For this review, take the finished solid that the model builds, in its own axes (mm). Give positions to 0.01 mm unless a question says otherwise; leave off trailing zeros. Write each loop counter-clockwise with the first axis right and the second up, starting at its lowest first coordinate (ties: lowest second). Pieces come first, ordered by that corner, then holes. Notation, with made-up numbers: (-31, -25.75) -> (27, -25.75) arc R29 cw to (27, -2.75) -> close; hole circle Ø3 at (60.5, 7). An arc over 180 degrees is marked (long way). Write item = value, one per line.
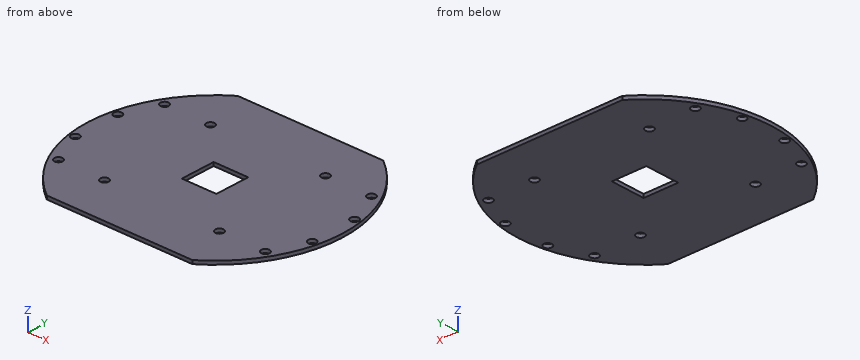
```python
from build123d import *

# Parameters (mm, degrees)
F1_DEPTH = 3
F3_D     = 7
F5_D     = 7
F6_W     = 30
F6_H     = 30
F7_DEPTH = 3.001


# Not quite as in the source:
# - a feature names something its author has since deleted; it is built from what else it names


with BuildPart() as f1:
    # F0 (on Top) → F1 (new body)
    with BuildSketch(Plane.XY):
        with BuildLine():
            Line((63.2455532034, 90), (-63.2455532034, 90))
            ThreePointArc((-63.2455532034, 90), (-110, 0), (-63.2455532034, -90))
            Line((-63.2455532034, -90), (63.2455532034, -90))
            ThreePointArc((63.2455532034, -90), (110, 0), (63.2455532034, 90))
        make_face()
    extrude(amount=F1_DEPTH)

    # F3 (through all)
    with Locations(Plane.XY.offset(3)):
        with Locations((-103, 20), (-103, -20), (-90, 50), (-90, -50), (90, -50), (90, 50), (103, 20), (103, -20)):
            Hole(F3_D / 2)

    # F5 (through all)
    with Locations(Plane.XY.offset(3)):
        with Locations((-50, 50), (50, 50), (50, -50), (-50, -50)):
            Hole(F5_D / 2)

    # F6 (on face) → F7 (cut, through all)
    with BuildSketch(Plane.XY.offset(3)):
        Rectangle(F6_W, F6_H)
    extrude(amount=-F7_DEPTH, mode=Mode.SUBTRACT)


solid = f1.part
```
(1) Take a section at B-B (x = 3.5). Write out the cut boundary in (y, z), plus the area to 3 significant figures.
Answers below:
outline = (-90, 0) -> (-15, 0) -> (-15, 3) -> (-90, 3) -> close; (15, 0) -> (90, 0) -> (90, 3) -> (15, 3) -> close
area = 450 mm^2
(2) Take a section at C-C (z = 0.85). Count the separate pieces of the cut face and the enclosed holes in it, plus the area to 3 significant figures.
Answers below:
separate_pieces = 1
enclosed_holes = 13
area = 33,200 mm^2
(3) Take a section at A-A (x = 90). Write out the cut boundary in (y, z), plus the area to 3 significant figures.
Answers below:
outline = (-63.25, 0) -> (-53.5, 0) -> (-53.5, 3) -> (-63.25, 3) -> close; (-46.5, 0) -> (46.5, 0) -> (46.5, 3) -> (-46.5, 3) -> close; (53.5, 0) -> (63.25, 0) -> (63.25, 3) -> (53.5, 3) -> close
area = 337 mm^2
(4) Take a section at D-D (y = 3). Write out the cut boundary in (x, z).
Answers below:
outline = (-109.96, 0) -> (-15, 0) -> (-15, 3) -> (-109.96, 3) -> close; (15, 0) -> (109.96, 0) -> (109.96, 3) -> (15, 3) -> close
(5) To check wall thickness, follow probe 1 along Y at (x, z) = (-50, 1.35); probe 2 along Y at (x, z) = (6.5, 2.3); probe 3 along X at (y, z) = (-48, 1.75). State the ranges of each line that lie inside material, in increasing order.
Answers below:
probe_1 = -90 to -53.5, -46.5 to 46.5, 53.5 to 90
probe_2 = -90 to -15, 15 to 90
probe_3 = -98.97 to -92.87, -87.13 to -52.87, -47.13 to 47.13, 52.87 to 87.13, 92.87 to 98.97
